from build123d import *

# Parameters (mm, degrees)
F0_W            = 71.5283732861
F0_H            = 64.1776323318
F1_DEPTH        = 89.916
F2_SIZE2        = 25.4
F2_SIZE         = 5.08
F5_DEPTH        = 135.128
F6_SIZE         = 5.08
F7_T            = -2.54
F9_D            = 5.5
F9_CBORE_D      = 6
F9_CBORE_DEPTH  = 1
F10_D           = 5.5
F10_CBORE_D     = 8
F10_CBORE_DEPTH = 1
F11_R           = 8
F12_R           = 8


with BuildPart() as f1:
    # F0 (on Front) → F1 (new body)
    with BuildSketch(Plane.XZ):
        with Locations((6.926660426, -4.6648941934)):
            Rectangle(F0_W, F0_H)
    extrude(amount=F1_DEPTH)

    # F2
    f2_edges = [f1.edges().sort_by_distance(p)[0] for p in [
        (42.690847, -44.958, 27.423922),
    ]]
    f2_side = f1.faces().sort_by_distance((6.92666, -44.958, 27.423922))[0]
    chamfer(f2_edges, length=F2_SIZE, length2=F2_SIZE2, reference=f2_side)


with BuildPart() as f5:
    # F4 (on Front) → F5 (new body)
    with BuildSketch(Plane.XZ):
        Polygon((40.32824561, 37.3740494251), (-64.0106573701, 33.7145887315), (-66.4161741734, -3.6638199817), (-23.4177149832, 0), (-23.4177149832, -41.7669005692), (40.32824561, -36.2140648067), align=None)
    extrude(amount=F5_DEPTH)

    # F6
    f6_edges = [f5.edges().sort_by_distance(p)[0] for p in [
        (-11.841206, -135.128, 35.544319),
    ]]
    chamfer(f6_edges, length=F6_SIZE)

    # F7
    f7_openings = [f5.faces().sort_by_distance(p)[0] for p in [
        (-3.73286, -135.128, 0.037818),
    ]]
    offset(amount=F7_T, openings=f7_openings, kind=Kind.INTERSECTION)

    # F9 (through all)
    with Locations(Plane(origin=(-1.2596562909, 0, 35.915443977), x_dir=(0.9993855151, 0, 0.0350512791), z_dir=(-0.0350512791, 0, 0.9993855151))):
        with Locations((-25.099163875, -58.0401532352)):
            CounterBoreHole(F9_D / 2, F9_CBORE_D / 2, F9_CBORE_DEPTH)

    # F10 (through all)
    with Locations(Plane(origin=(-1.2596562909, 0, 35.915443977), x_dir=(0.9993855151, 0, 0.0350512791), z_dir=(-0.0350512791, 0, 0.9993855151))):
        with Locations((15.1631087065, -84.5927745104)):
            CounterBoreHole(F10_D / 2, F10_CBORE_D / 2, F10_CBORE_DEPTH)

    # F11
    f11_edges = [f5.edges().sort_by_distance(p)[0] for p in [
        (-11.841206, 0, 35.544319),
    ]]
    fillet(f11_edges, radius=F11_R)

    # F12
    f12_edges = [f5.edges().sort_by_distance(p)[0] for p in [
        (40.328246, -67.564, -36.214065),
    ]]
    fillet(f12_edges, radius=F12_R)


solid = f5.part
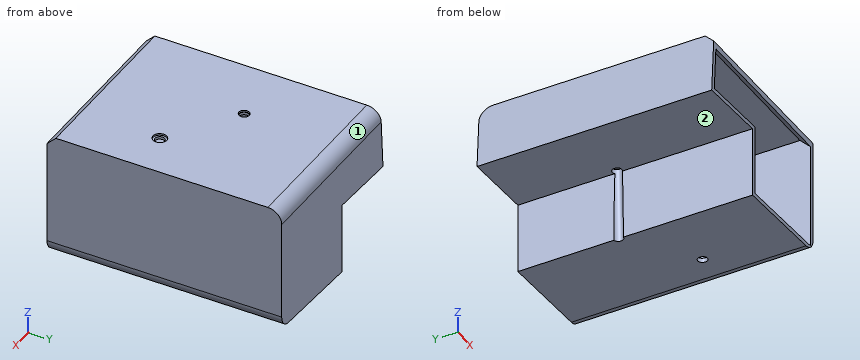
Model file for the job. Use its own axes, mm. Face numbers are marked on the shaded views. A direction names the side the tool comes from. Coordinates: 2 decimals unless noted, no trailing zeros. Order: outer loops, then holes, each group sorted by start corner. A loop starts at its lowest first (then second) coordinate and runs counter-clockwise, first axis right, second up. Notation, with made-up numbers: M -2,74.5 L 43,74.5 A19 cw 43,96.5 Z; hole C -24.75,-33.75 d9. An arc over 180 degrees is marked long. Return JSON: item names as keys, results as strings.
1. Tool access for the marked faces 1 and 2: list every direction of +Z, -Z, +X, -X, +Y, -Y with a clear straight run to the whole face (end or side of a thin tool).
Ans:
{"face 1": "+Z, -X, +Y", "face 2": "-Z, +Y, -Y"}
2. Saw through at A-A (y = -49). Give the cut face in (x, z).
Ans:
{"outline": "M -66.42,-3.66 L -23.42,0 L -23.42,-41.77 L 33.02,-36.85 A8 ccw 40.33,-28.88 L 40.33,37.37 L -64.01,33.71 Z; hole M -63.69,-0.88 L -20.88,2.77 L -20.88,-39 L 37.79,-33.89 L 37.79,34.74 L -61.62,31.26 Z"}
3. Drill centre lines: probe 1 along X at (y, z) = (-118.5, -23.5); probe 2 along X at (y, z) = (-36.5, 25.5); probe 3 along Y at (x, z) = (-10, -15). Where is each one in solid material? Low to high.
Ans:
{"probe 1": "-23.42 to -20.88, 37.79 to 40.33", "probe 2": "-64.54 to -61.99, 37.79 to 40.33", "probe 3": "-2.54 to 0"}
4. Saw through at B-B (z = 17.5). Give the cut face in (x, y).
Ans:
{"outline": "M -65.05,-135.13 L -62.51,-135.13 L -62.51,-2.54 L 37.79,-2.54 L 37.79,-135.13 L 40.33,-135.13 L 40.33,0 L -65.05,0 Z"}
5. Flat gauge pins, fed straight in: pin 1 (8 mm diameter, centred on y = -39.5, z = 28, fed in from -X); pin 2 (1.5 mm diameter, centred on x = 17.5, y = -72.5, fed in from +Z); pin 3 (21 mm diameter, centred on y = -87.5, z = -23.5, fed in from -X). Where does each tip first touch, or does it go through?
Ans:
{"pin 1": "x = -64.64", "pin 2": "z = 36.6", "pin 3": "x = -23.42"}
